from build123d import *

# Parameters (mm, degrees)
SKETCH1_W               = 105.991744741
SKETCH1_H               = 29.109935465
BOSS_EXTRUDE1_DEPTH     = 84
CUT_EXTRUDE1_DEPTH      = 199.997997189
CUT_EXTRUDE1_DEPTH_BACK = 3
SKETCH3_W               = 15.49999237
SKETCH3_H               = 11.5
CUT_EXTRUDE2_DEPTH      = 139.309528443
CUT_EXTRUDE2_DEPTH_BACK = 139.309528443
SKETCH4_W               = 27.109935465
SKETCH4_H               = 78
SKETCH5_W               = 9.5
SKETCH5_H               = 11.499607086
SKETCH5_W_2             = 18.49999237
SKETCH5_H_2             = 9.868988037
SKETCH5_H_3             = 7.550139481
SKETCH5_W_3             = 15.472055618
SKETCH5_H_4             = 19.899999618
SKETCH5_W_4             = 15.574996948
SKETCH5_H_5             = 22.25664711
SKETCH5_W_5             = 16.499984741
SKETCH5_H_6             = 14.249998093
SKETCH5_W_6             = 9
SKETCH5_H_7             = 3
CUT_EXTRUDE3_DEPTH      = 3
BOSS_EXTRUDE2_DEPTH     = 105.991744742
SKETCH7_R               = 1
CUT_EXTRUDE4_DEPTH      = 199.99799719
LPATTERN1_COUNT         = 28
LPATTERN1_PITCH         = 3.71


with BuildPart() as part:
    # Sketch1 → Boss-Extrude1 (new body)
    with BuildSketch(Plane(origin=(0, 0, 0), x_dir=(1, 0, 0), z_dir=(0, 1, 0))):
        with Locations((125.062902141, -14.415287787)):
            Rectangle(SKETCH1_W, SKETCH1_H)
    extrude(amount=BOSS_EXTRUDE1_DEPTH)

    # Sketch3 → Cut-Extrude1 (cut, two sides: drawn at the far end of the back side and taken through both)
    with BuildSketch(Plane(origin=(0, 84, 0), x_dir=(1, 0, 0), z_dir=(0, 1, 0)).offset(-CUT_EXTRUDE1_DEPTH_BACK)):
        with Locations((117.700000763, -7.750003815)):
            Rectangle(SKETCH3_W, SKETCH3_H)
    extrude(amount=CUT_EXTRUDE1_DEPTH + CUT_EXTRUDE1_DEPTH_BACK, mode=Mode.SUBTRACT)

    # Sketch4 → Cut-Extrude2 (cut, two sides: drawn at the far end of the back side and taken through both)
    with BuildSketch(Plane.ZY.offset(-72.06702977).offset(-CUT_EXTRUDE2_DEPTH_BACK)):
        with Locations((15.415287787, 42)):
            Rectangle(SKETCH4_W, SKETCH4_H)
    extrude(amount=CUT_EXTRUDE2_DEPTH + CUT_EXTRUDE2_DEPTH_BACK, mode=Mode.SUBTRACT)

    # Sketch5 → Cut-Extrude3 (cut)
    with BuildSketch(Plane.XZ):
        with Locations((81.127942856, 11.617159806)):
            Rectangle(SKETCH5_W, SKETCH5_H)
        with Locations((99.027940567, 21.182469331)):
            Rectangle(SKETCH5_W_2, SKETCH5_H_2)
        with Locations((99.027940567, 9.992033472)):
            Rectangle(SKETCH5_W_2, SKETCH5_H_3)
        with Locations((117.713969139, 16.16696354)):
            Rectangle(SKETCH5_W_3, SKETCH5_H_4)
        with Locations((134.662498474, 14.988639794)):
            Rectangle(SKETCH5_W_4, SKETCH5_H_5)
        with Locations((152.049995423, 13.481646538)):
            Rectangle(SKETCH5_W_5, SKETCH5_H_6)
        with Locations((167.149993896, 7.507040024)):
            Rectangle(SKETCH5_W_6, SKETCH5_H_7)
    extrude(amount=-CUT_EXTRUDE3_DEPTH, mode=Mode.SUBTRACT)

    # Sketch6 → Boss-Extrude2 (add)
    with BuildSketch(Plane.ZY.offset(-72.06702977)):
        Polygon((-0.139679946, 33), (-0.139679946, 51), (-4.229633498, 53.254147276), (-7.960635886, 51), (-7.960635886, 33), (-4.229633498, 30.638664216), align=None)
    extrude(amount=-BOSS_EXTRUDE2_DEPTH)

    # Sketch7 → Cut-Extrude4 (cut, symmetric)
    with BuildSketch(Plane(origin=(0, 0, 0), x_dir=(1, 0, 0), z_dir=(0, 1, 0))):
        with Locations(Location((75.77702977, 2.239679946, 0), (0, 0, 90))):
            Circle(SKETCH7_R)
    cut_extrude4 = extrude(amount=CUT_EXTRUDE4_DEPTH, both=True, mode=Mode.SUBTRACT)

    # LPattern1: Cut-Extrude4 ×28
    with Locations(*[(i * LPATTERN1_PITCH, 0, 0) for i in range(1, LPATTERN1_COUNT)]):
        add(cut_extrude4, mode=Mode.SUBTRACT)


solid = part.part
Here's how the part is built. I have some questions about the finished solid (model axes, mm). A direction names the side the tool comes from. Coordinates: 2 decimals unless noted, no trailing zeros. Order: outer loops, then holes, each group sorted by start corner. A loop starts at its lowest first (then second) coordinate and runs counter-clockwise, first axis right, second up. Notation, with made-up numbers: M 54.5,64.5 L 70.5,64.5 A25 cw 70.5,80.5 Z; hole C 75.25,-6 d4. An arc over 180 degrees is marked long. Answer as CSV lines item,"result".
Item 1: Imagine slicing it at A-A on z = 11.5. Give the number of separate pieces and of enclosed holes in the cut face, plus the area to 3 significant figures.
Results found:
separate pieces,"8"
enclosed holes,"0"
area,"363 mm2"
Item 2: Imagine slicing it at C-C on y = 58. Write out the boundary of the cut face in (x, z), plus the area to 3 significant figures.
Results found:
outline,"M 72.07,-0.14 L 178.06,-0.14 L 178.06,1.86 L 72.07,1.86 Z"
area,"212 mm2"
Item 3: We'd pull the mould along X, two halves only. Please class faces 1 (the face through (72.067, 42, 1)), 2 (the face through (124, 16, -0.14)), 3 (the face through (143.8, 1, 13)): +X half, -X half, draft (parallel to the pull), parting line (faces both ways), or undercut.
Results found:
face 1,"-X half"
face 2,"draft"
face 3,"undercut"
Item 4: If I drill on line 1 (Y direction, x = 76, z = 24); line 2 (Z direction, x = 169, y = 46); line 3 (Z direction, x = 109, y = 75.5), over which ranges is the centre line in solid material (lowest first)?
Results found:
line 1,"0 to 3, 81 to 84"
line 2,"-7.96 to -3.12, -1.36 to 1.86"
line 3,"-0.14 to 1.86"
Item 5: For pin 1 (12 mm diameter, centred on x = 138.5, y = 14.5, fed in from +Z); pin 2 (3.5 mm diameter, centred on x = 94.5, y = 1.5, fed in from -Z); pin 3 (3 mm diameter, centred on x = 131.43, z = -2.24, fed in from -Y), each with a flat end and sliding along its axis, tell me the tip position at first contact or that it passes through.
Results found:
pin 1,"z = 1.86"
pin 2,"z = -0.14"
pin 3,"y = 30.92"
Item 6: On a 3-axis mill with a long thin cutter (end or side, diameter ignored), from which of +Z, -Z, +X, -X, +Y, -Y can I reach the whole of each face in a straight line? I mean faces 4 (the face through (118, 82, 13.5)), 5 (the face through (124, 0, 5)), 6 (the face through (85.878, 1, 12)). Say none if no direction works.
Results found:
face 4,"+Y, -Y"
face 5,"+Z, -Z, +X, -X, -Y"
face 6,"-Y"
